Study the drawing (mm; zero at the part's minimum x, y, z) and answer. A direction names the side the tool comes from. Round coordinates to 2 decimals unless told otherwise and drop trailing zeros. Loops run counter-clockwise (first coordinate to the right, second up) from the corner with the lowest first, then second, coordinate; pieces in that order, holes last. Notation, with made-up numbers: M 15,85.5 L 23,85.5 A35 cw 23,121.5 Z; hole C 71,65.5 d4. An arc over 180 degrees is marked long. Put each result on its own line as item: value. Start each with the question number.
(1) Section A-A, the plane z = 11.25 is taken. Determine the outline of the cut face in (x, y).
(2) Which of the six approach directions +Z, -Z, +X, -X, +Y, -Y give full straight-line access (tool end or side, diameter ignored) to the marked faces 1, 2 and 3?
(3) Straight lines are drawn through the part: line 1 (Y direction, x = 18, z = 7); line 2 (X direction, y = 15, z = 2). For each, find the intervals that lie inside material, in ascending order.
(4) Section C-C, the plane x = 17 is taken. Determine the outline of the cut face in (y, z).
(5) A flat-ended cylindrical pin translates along its axis: P1, Ø7.5, axis at x = 9, z = 9, coming from the -Y side. Find the tip coordinate at first contact, or state that the pin passes through.
(6) Section B-B, the plane y = 16.5 is taken. Determine the outline of the cut face in (x, z), then the cut area to 3 significant figures.
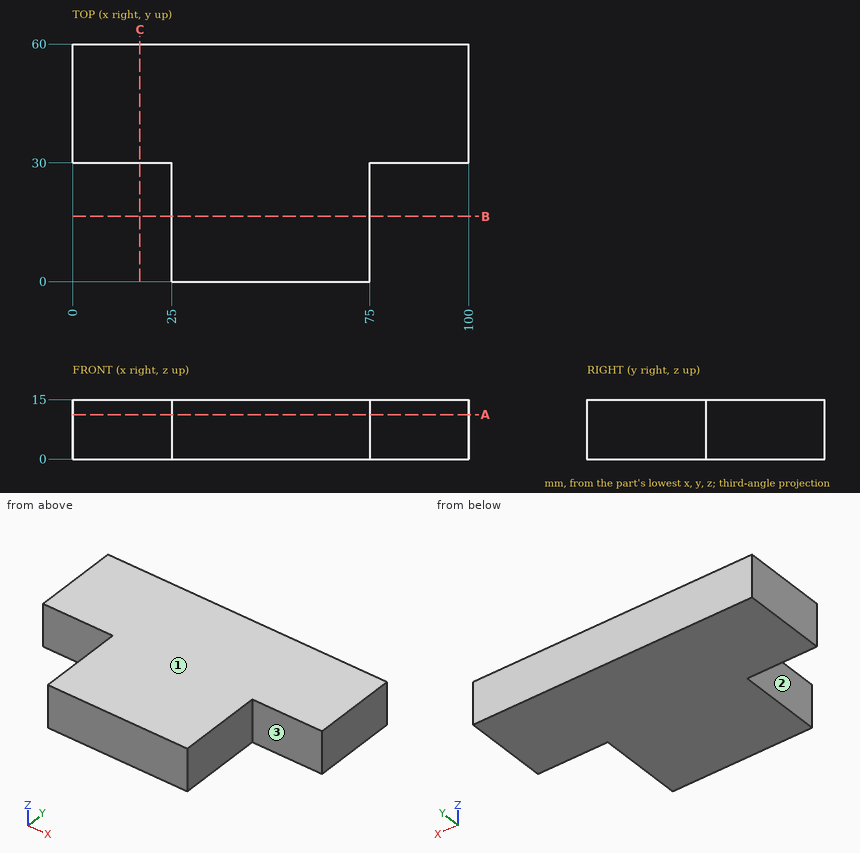
Recorded:
1. outline: M 0,30 L 25,30 L 25,0 L 75,0 L 75,30 L 100,30 L 100,60 L 0,60 Z
2. face 1: +Z, +X, -X, +Y, -Y
2. face 2: +Z, -Z, -X, -Y
2. face 3: +Z, -Z, +X, -Y
3. line 1: y = 30 to 60
3. line 2: x = 25 to 75
4. outline: M 30,0 L 60,0 L 60,15 L 30,15 Z
5. P1: stops at y = 30
6. outline: M 25,0 L 75,0 L 75,15 L 25,15 Z
6. area: 750 mm²
